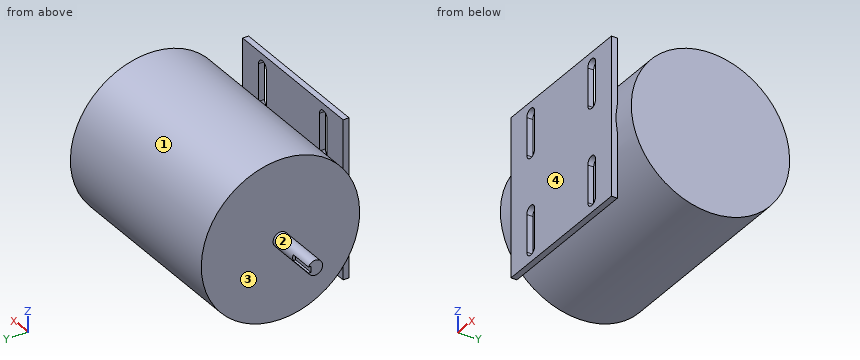
from build123d import *

# Parameters (mm, degrees)
CROQUIS1_R              = 85
SALIENTE_EXTRUIR1_DEPTH = 215
CROQUIS2_R              = 7.9375
SALIENTE_EXTRUIR2_DEPTH = 57.15
CROQUIS4_W              = 165
CROQUIS4_H              = 170
SALIENTE_EXTRUIR3_DEPTH = 6.35
CORTAR_EXTRUIR1_DEPTH   = 25
CORTAR_EXTRUIR2_DEPTH   = 10


with BuildPart() as part:
    # Croquis1 → Saliente-Extruir1 (new body)
    with BuildSketch(Plane(origin=(0, 0, 0), x_dir=(0, 0, -1), z_dir=(1, 0, 0))):
        Circle(CROQUIS1_R)
    extrude(amount=SALIENTE_EXTRUIR1_DEPTH)

    # Croquis2 → Saliente-Extruir2 (add)
    with BuildSketch(Plane.ZY):
        Circle(CROQUIS2_R)
    extrude(amount=SALIENTE_EXTRUIR2_DEPTH)

    # Croquis4 → Saliente-Extruir3 (add)
    with BuildSketch(Plane(origin=(0, -90, 0), x_dir=(1, 0, 0), z_dir=(0, 1, 0))):
        with Locations((107.5, 0)):
            Rectangle(CROQUIS4_W, CROQUIS4_H)
    extrude(amount=SALIENTE_EXTRUIR3_DEPTH)

    # Croquis5 → Cortar-Extruir1 (cut)
    with BuildSketch(Plane.ZY.offset(57.15)):
        with BuildLine():
            Line((-3.175, 7.274838916), (-3.175, 4.7625))
            Line((-3.175, 4.7625), (3.175, 4.7625))
            Line((3.175, 4.7625), (3.175, 7.274838916))
            ThreePointArc((3.175, 7.274838916), (0, 7.9375), (-3.175, 7.274838916))
        make_face()
    extrude(amount=-CORTAR_EXTRUIR1_DEPTH, mode=Mode.SUBTRACT)

    # Croquis7 → Cortar-Extruir2 (cut)
    with BuildSketch(Plane.XZ.offset(90)):
        with BuildLine():
            Line((51.15, 71.515151515), (51.15, 31.515151515))
            ThreePointArc((51.15, 31.515151515), (57.5, 25.165151515), (63.85, 31.515151515))
            Line((63.85, 31.515151515), (63.85, 71.515151515))
            ThreePointArc((63.85, 71.515151515), (57.5, 77.865151515), (51.15, 71.515151515))
        make_face()
        with BuildLine():
            Line((151.15, 71.515151515), (151.15, 31.515151515))
            ThreePointArc((151.15, 31.515151515), (157.5, 25.165151515), (163.85, 31.515151515))
            Line((163.85, 31.515151515), (163.85, 71.515151515))
            ThreePointArc((163.85, 71.515151515), (157.5, 77.865151515), (151.15, 71.515151515))
        make_face()
        with BuildLine():
            Line((51.15, -31.515151515), (51.15, -71.515151515))
            ThreePointArc((51.15, -71.515151515), (57.5, -77.865151515), (63.85, -71.515151515))
            Line((63.85, -71.515151515), (63.85, -31.515151515))
            ThreePointArc((63.85, -31.515151515), (57.5, -25.165151515), (51.15, -31.515151515))
        make_face()
        with BuildLine():
            Line((151.15, -31.515151515), (151.15, -71.515151515))
            ThreePointArc((151.15, -71.515151515), (157.5, -77.865151515), (163.85, -71.515151515))
            Line((163.85, -71.515151515), (163.85, -31.515151515))
            ThreePointArc((163.85, -31.515151515), (157.5, -25.165151515), (151.15, -31.515151515))
        make_face()
    extrude(amount=-CORTAR_EXTRUIR2_DEPTH, mode=Mode.SUBTRACT)


solid = part.part
Could you check a few things on this model? Use its own coordinates, in mm. Face numbers are marked on the shaded views. Give positions to 0.01 mm unless a question says otherwise; leave off trailing zeros. Order: outer loops, then holes, each group sorted by start corner. A loop starts at its lowest first (then second) coordinate and runs counter-clockwise, first axis right, second up. Notation, with made-up numbers: M 72,18.25 L 83,18.25 A15 cw 83,35.25 Z; hole C 26.25,72 d5. An arc over 180 degrees is marked long. One line per question, with ' | ' between items.
1. I want a section at C-C (y = 0). List the corners of the cut face in (x, z) for me.
Results:
outline: M -57.15,-7.94 L 0,-7.94 L 0,-85 L 215,-85 L 215,85 L 0,85 L 0,7.94 L -57.15,7.94 Z
2. I want a section at B-B (z = 59). List the corners of the cut face in (x, y) for me.
Results:
outline: M 0,-61.19 L 215,-61.19 L 215,61.19 L 0,61.19 Z; M 25,-90 L 51.15,-90 L 51.15,-83.65 L 25,-83.65 Z; M 63.85,-90 L 151.15,-90 L 151.15,-83.65 L 63.85,-83.65 Z; M 163.85,-90 L 190,-90 L 190,-83.65 L 163.85,-83.65 Z
3. I want a section at D-D (z = 0). List the corners of the cut face in (x, y) for me.
Results:
outline: M -57.15,-7.94 L 0,-7.94 L 0,-85 L 25,-85 L 25,-90 L 190,-90 L 190,-85 L 215,-85 L 215,85 L 0,85 L 0,7.94 L -32.15,7.94 L -32.15,4.76 L -57.15,4.76 Z
4. We'd pull the mould along Y, two halves only. Please class the marked faces 1, 2, 3 and 4: +Y half, -Y half, draft (parallel to the pull), parting line (faces both ways), or undercut.
Results:
face 1: undercut | face 2: parting line | face 3: draft | face 4: -Y half
5. I'm going to push flat-ended pins straight in: pin 1 (1.9 mm diameter, centred on y = -88.5, z = 53.5, fed in from +X); pin 2 (8 mm diameter, centred on x = 115.5, y = -26, fed in from +Z); pin 3 (4 mm diameter, centred on y = -58, z = 3.5, fed in from -X). Where does each tip first touch, or does it pass through?
Results:
pin 1: x = 190 | pin 2: z = 82.1 | pin 3: x = 0
6. I want a section at A-A (x = 157.5). List the corners of the cut face in (y, z) for me.
Results:
outline: M -90,-85 L -83.65,-85 L -83.65,-77.87 L -90,-77.87 Z; M -90,-25.17 L -83.65,-25.17 L -83.65,-15.09 A85 ccw -81.19,-25.17 L -80,-25.17 L -80,-28.72 A85 ccw long -80,28.72 L -80,25.17 L -81.19,25.17 A85 ccw -83.65,15.09 L -83.65,25.17 L -90,25.17 Z; M -90,77.87 L -83.65,77.87 L -83.65,85 L -90,85 Z
7. If I drill on line 1 (Y direction, x = 127, z = -73); line 2 (X direction, y = -79, z = -20); line 3 (Z direction, x = 117, y = 34), over which ranges is the centre line in solid material (lowest first)?
Results:
line 1: -90 to -83.65, -43.54 to 43.54 | line 2: 0 to 215 | line 3: -77.9 to 77.9
